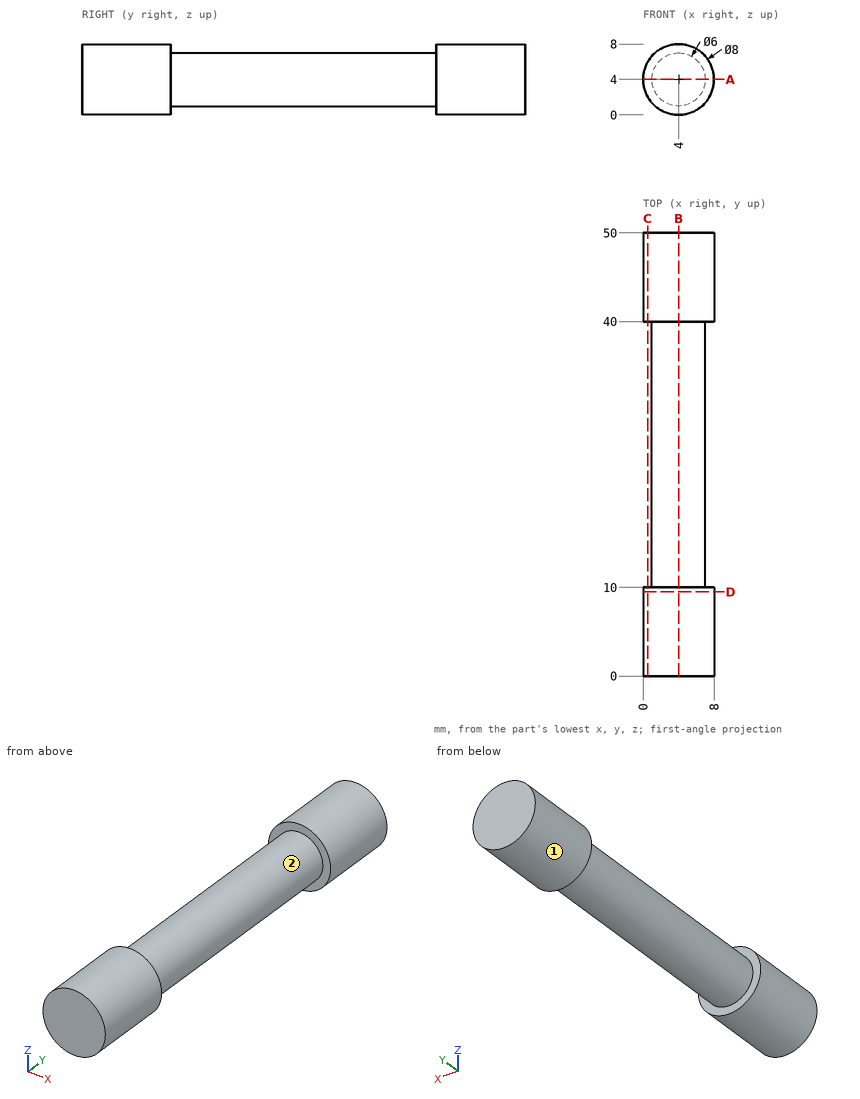
Check sheet for the drawn part. Datum: minimum x, y, z corner. Units: mm. A direction names the side the tool comes from. Give positions to 0.01 mm unless a question says otherwise; leave off trailing zeros. Order: outer loops, then holes, each group sorted by start corner. A loop starts at its lowest first (then second) coordinate and runs counter-clockwise, first axis right, second up. Notation, with made-up numbers: (4, 8.5) -> (49, 8.5) arc R14 ccw to (49, 13.5) -> close; hole circle Ø3 at (29, 59.5). An arc over 180 degrees is marked (long way). Return JSON: item names as keys, results as strings.
1. Cross-section at A-A, the plane z = 4. Record the cut outline in (x, y), plus the area to 3 significant figures.
From the geometry:
{"outline": "(0, 0) -> (8, 0) -> (8, 10) -> (7, 10) -> (7, 40) -> (8, 40) -> (8, 50) -> (0, 50) -> (0, 40) -> (1, 40) -> (1, 10) -> (0, 10) -> close", "area": "340 mm^2"}
2. Cross-section at C-C, the plane x = 0.5. Record the cut outline in (y, z), plus the area to 3 significant figures.
From the geometry:
{"outline": "(0, 2.06) -> (10, 2.06) -> (10, 5.94) -> (0, 5.94) -> close; (40, 2.06) -> (50, 2.06) -> (50, 5.94) -> (40, 5.94) -> close", "area": "77.5 mm^2"}
3. Set-up check for the marked faces 1 and 2: record each of +Z, -Z, +X, -X, +Y, -Y from which the full face is reachable in a straight line by a thin tool's end or side.
From the geometry:
{"face 1": "+Y, -Y", "face 2": "none"}
4. Cross-section at D-D, the plane y = 9.5. Record the cut outline in (x, z).
From the geometry:
{"outline": "circle Ø8 at (4, 4)"}
5. Cross-section at B-B, the plane x = 4. Record the cut outline in (y, z).
From the geometry:
{"outline": "(0, 0) -> (10, 0) -> (10, 1) -> (40, 1) -> (40, 0) -> (50, 0) -> (50, 8) -> (40, 8) -> (40, 7) -> (10, 7) -> (10, 8) -> (0, 8) -> close"}
6. Material ranges on probe 1 along Y at (x, z) = (4.75, 7.25); probe 2 along X at (y, z) = (10.5, 4.25); probe 3 along Z at (x, y) = (3.75, 42), recorded low to high. Write a range as [from, to].
From the geometry:
{"probe 1": "[0, 10], [40, 50]", "probe 2": "[1.01, 6.99]", "probe 3": "[0.01, 7.99]"}
7. Go/stop test with flat-tipped pins: P1, Ø1, axis at x = 6.5, z = 4.5, coming from the -Y side; P2, Ø2, axis at x = 6.5, y = 25.5, coming from the +Z side. Record where each tip stops, or that it passes through.
From the geometry:
{"P1": "y = 0", "P2": "z = 6.6"}
